Here's how the part is built. I have some questions about the finished solid (model axes, mm). Face numbers are marked on the shaded views. A direction names the side the tool comes from. Round coordinates to 2 decimals unless told otherwise and drop trailing zeros. Write each loop counter-clockwise with the first axis right and the second up, starting at its lowest first coordinate (ties: lowest second). Pieces come first, ordered by that corner, then holes. Notation, with made-up numbers: (57, 21) - (76, 21) arc R21 ccw to (76, 55) - close; hole circle Ø10 at (28, 6.5). An arc over 180 degrees is marked (long way). Return JSON: item names as keys, results as strings. Group by question number.
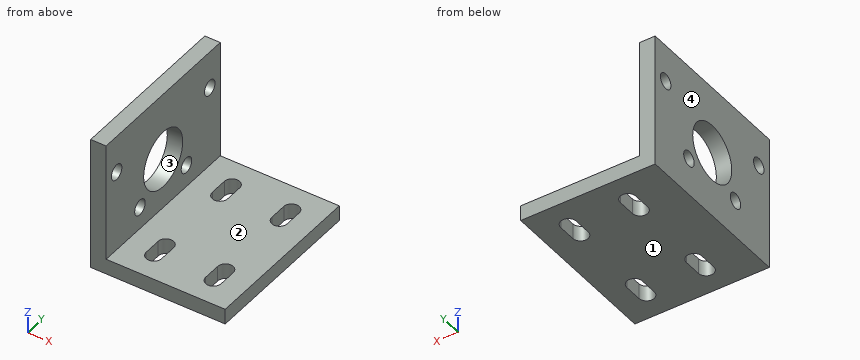
Autodesk Fusion 360 part; units mm, degrees
sketch "Sketch1" plane through (0, 0, 0) normal (0, 1, 0) x (1, 0, 0) in component "Component"
  line L0 (0, 0) -> (30.5, 0)
  line L1 (0, 0) -> (0, -30.5)
  line L2 (30.5, 0) -> (30.5, -3.5)
  line L3 (0, -30.5) -> (3.5, -30.5)
  line L4 (3.5, -30.5) -> (3.5, -3.5)
  line L5 (3.5, -3.5) -> (30.5, -3.5)
  dimension "d3" = 3.5
  dimension "d4" = 3.5
  dimension "d24" = 27
  dimension "d25" = 27
extrude "Extrude1" add sketch "Sketch1" along normal blind 38 in component "Component"
sketch "Sketch2" plane through (3.5, 0, 0) normal (1, 0, 0) x (0, 1, 0) in component "Component"
  line L0 (0, 30.5) -> (0, 3.5)
  line L1 (0, 3.5) -> (38, 3.5)
  line L2 (38, 3.5) -> (38, 30.5)
  line L3 (38, 30.5) -> (0, 30.5)
sketch "Sketch3" plane through (0, 0, 3.5) normal (0, 0, 1) x (-1, 0, 0) in component "Component"
  line L0 (-3.5, 0) -> (-30.5, 0)
  line L1 (-30.5, 0) -> (-30.5, -38)
  line L2 (-3.5, 0) -> (-3.5, -38) construction
  line L3 (-3.5, -19) -> (-10.25, -19) construction
  line L4 (-3.5, -38) -> (-3.5, 0) construction
  line L5 (0, 0) -> (0, -38) construction
  line L6 (-10.25, -19) -> (-10.25, -28) construction
  line L7 (-10.25, -28) -> (-23.75, -28) construction
  line L8 (-10.25, -28) -> (-10.25, -32) construction
  line L9 (-10.25, -32) -> (-8.5, -32) construction
  line L10 (-10.25, -28) -> (-8.5, -28) construction
  arc A0 (-12, -32) -> (-8.5, -32) centre (-10.25, -32) ccw
  arc A1 (-8.5, -28) -> (-12, -28) centre (-10.25, -28) ccw
  line L11 (-8.5, -28) -> (-8.5, -32)
  line L12 (-12, -28) -> (-12, -32)
  line L13 (-22, -28) -> (-22, -32)
  arc A2 (-22, -28) -> (-25.5, -28) centre (-23.75, -28) ccw
  line L14 (-25.5, -28) -> (-25.5, -32)
  arc A3 (-25.5, -32) -> (-22, -32) centre (-23.75, -32) ccw
  line L15 (-8.5, -10) -> (-8.5, -6)
  arc A4 (-12, -10) -> (-8.5, -10) centre (-10.25, -10) ccw
  line L16 (-12, -10) -> (-12, -6)
  arc A5 (-8.5, -6) -> (-12, -6) centre (-10.25, -6) ccw
  line L17 (-22, -10) -> (-22, -6)
  arc A6 (-25.5, -10) -> (-22, -10) centre (-23.75, -10) ccw
  line L18 (-25.5, -10) -> (-25.5, -6)
  arc A7 (-22, -6) -> (-25.5, -6) centre (-23.75, -6) ccw
  dimension "d27" = 6.75
  dimension "d28" = 9
  dimension "d29" = 13.5
  dimension "d30" = 4
  dimension "d31" = 1.75
  dimension "d34" = -13.5
  dimension "d35" = 0
extrude "Extrude3" cut sketch "Sketch3" against normal through all in component "Component"
sketch "Sketch2 (2)" plane through (3.5, 0, 0) normal (1, 0, 0) x (0, 1, 0)
  line L0 (0, 30.5) -> (0, 3.5) construction
  line L1 (0, 3.5) -> (38, 3.5) construction
  line L2 (38, 3.5) -> (38, 30.5) construction
  line L3 (38, 30.5) -> (0, 30.5) construction
  line L4 (19, 3.5) -> (19, 15) construction
  circle A0 centre (19, 15) radius 6.5
  line L5 (19, 15) -> (19, 22) construction
  line L6 (19, 22) -> (3.5, 22) construction
  circle A1 centre (3.5, 22) radius 1.75
  line L7 (19, 22) -> (11.25, 8.5766) construction
  circle A2 centre (11.25, 8.5766) radius 1.75
  circle A3 centre (34.5, 22) radius 1.75
  circle A4 centre (26.75, 8.5766) radius 1.75
  dimension "d37" = 11.5
  dimension "d38" = 13
  dimension "d39" = 7
  dimension "d40" = 15.5
  dimension "d41" = 3.5
  dimension "d42" = 60
  dimension "d43" = 3.5
extrude "Extrude4" cut sketch "Sketch2 (2)" against normal through all in component "Component"
component "Component" placed x (1, 0, 0) y (0, 1, 0) z (0, 0, 1) at (0, 0, 0)
equation "d25 = d24"
equation "d28 = ( 18 / 2 ) * 1 mm"
equation "d31 = ( 3.5 / 2 ) * 1 mm"
equation "d40 = ( 31 / 2 ) * 1 mm"
equation "d42 = ( 360 / 6 ) * 1 deg"
equation "d43 = d41"
1) I need wall thicknesses on line 1 along Z through (x, y) = (1, 19); line 2 along Z through (x, y) = (2.15, 26.75); line 3 along Y through (x, z) = (2, 9). Which ranges of each line are inside material? Lowest first, please.
2) Imagine slicing it at B-B (x = 23.75). Please give me the cut outline in (y, z).
3) For the marked faces 1 and 2, which set-ups out of +Z, -Z, +X, -X, +Y, -Y let a thin tool reach every point of the face, with its end or its side?
4) Will these pins go through, and if not, where does the flat tip stop? pin 1 Ø8 at (x, y) = (17.5, 23) entering from +Z; pin 2 Ø3 at (y, z) = (13, 14.5) entering from +X.
5) Imagine slicing it at D-D (y = 17.5). Please give me the cut outline in (x, z), plus the area to 3 significant figures.
6) Imagine slicing it at A-A (y = 6.5). Please give me the cut outline in (x, z), plus the area to 3 significant figures.
7) If we mould it in two halves opening along Y, with no side actions, what happens to the marked faces 3 and 4? For each: released by +Y, released by -Y, zero draft, split by the parting line, or undercut.
8) Imagine slicing it at C-C (z = 22). Please give me the cut outline in (x, y), plus the area to 4 significant figures.
Results found:
{
 "1": {"line 1": "z = 0 to 8.5, 21.5 to 30.5", "line 2": "z = 0 to 6.83, 10.33 to 30.5", "line 3": "y = 0 to 9.55, 12.95 to 16.5, 21.5 to 25.05, 28.45 to 38"},
 "2": {"outline": "(0, 0) - (4.25, 0) - (4.25, 3.5) - (0, 3.5) - close; (11.75, 0) - (26.25, 0) - (26.25, 3.5) - (11.75, 3.5) - close; (33.75, 0) - (38, 0) - (38, 3.5) - (33.75, 3.5) - close"},
 "3": {"face 1": "-Z, +X, -X, +Y, -Y", "face 2": "+Z, +X, +Y, -Y"},
 "4": {"pin 1": "stops at z = 3.5", "pin 2": "stops at x = 3.5"},
 "5": {"outline": "(0, 0) - (30.5, 0) - (30.5, 3.5) - (3.5, 3.5) - (3.5, 8.68) - (0, 8.68) - close; (0, 21.32) - (3.5, 21.32) - (3.5, 30.5) - (0, 30.5) - close", "area": "157 mm²"},
 "6": {"outline": "(0, 0) - (8.5, 0) - (8.5, 3.5) - (3.5, 3.5) - (3.5, 30.5) - (0, 30.5) - close; (12, 0) - (22, 0) - (22, 3.5) - (12, 3.5) - close; (25.5, 0) - (30.5, 0) - (30.5, 3.5) - (25.5, 3.5) - close", "area": "177 mm²"},
 "7": {"face 3": "undercut", "face 4": "zero draft"},
 "8": {"outline": "(0, 0) - (3.5, 0) - (3.5, 1.75) - (0, 1.75) - close; (0, 5.25) - (3.5, 5.25) - (3.5, 32.75) - (0, 32.75) - close; (0, 36.25) - (3.5, 36.25) - (3.5, 38) - (0, 38) - close", "area": "108.5 mm²"}
}
